The figure shows three views and two pictorial views of one solid part (mm, origin at its lowest corner). Answer the questions. Coordinates: 2 decimals unless noted, no trailing zeros. Write each loop counter-clockwise with the first axis right and the second up, starting at its lowest first coordinate (ties: lowest second). Pieces come first, ordered by that corner, then holes.
Item 1: Section B-B (z = 92) is taken. Give the vertices of the cut face in (x, y) (1 decimal).
Item 2: Each of these flat-tipped pins is pushed along its axis until it touches: P1, Ø3, axis at y = 7.5, z = 244, coming from the +X side; P2, Ø5, axis at y = 2, z = 206, coming from the -X side. Where does it stop, or does it pass through?
Item 3: Section A-A (y = 5.75) is taken. Give the vertices of the cut face in (x, z), then the cut area to 3 significant figures.
Item 4: Straight lines are drawn through the part: probe 1 along X at (y, z) = (7.75, 27.5); probe 2 along X at (y, z) = (7.25, 151). For each, find the intervals that lie inside material, in ascending order.
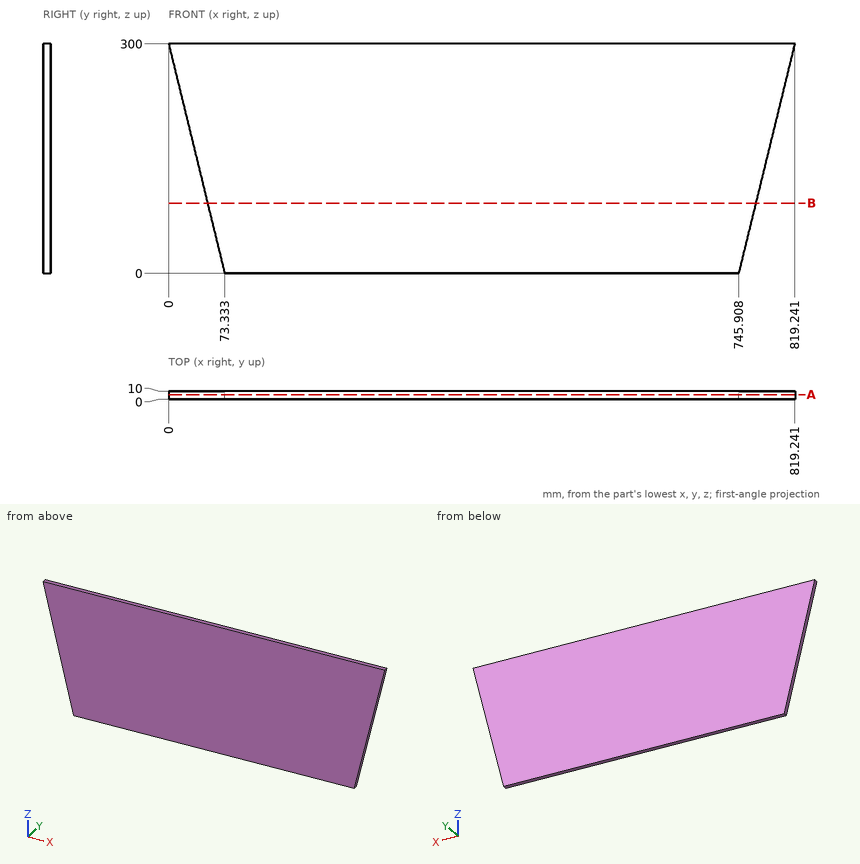
Established:
1. outline: (50.8, 0) - (768.4, 0) - (768.4, 10) - (50.8, 10) - close
2. P1: stops at x = 805.92
2. P2: stops at x = 22.37
3. outline: (0, 300) - (73.33, 0) - (745.91, 0) - (819.24, 300) - close
3. area: 224,000 mm2
4. probe 1: x = 66.61 to 752.63
4. probe 2: x = 36.42 to 782.82
